Build history of the part. All positions in model axes, mm. A direction names the side the tool comes from. Give positions to 0.01 mm unless a question says otherwise; leave off trailing zeros. Loops run counter-clockwise (first coordinate to the right, second up) from the corner with the lowest first, then second, coordinate; pieces in that order, holes last. Notation, with made-up numbers: (45, 20) - (92, 20) arc R21 ccw to (92, 49) - close; hole circle Ø8 at (-4, -36.5). An arc over 180 degrees is marked (long way). Return JSON: item names as keys, results as strings. Group by question number.
1) Slice it at D-D (x = 4.5). List the corners of the cut face in (y, z), and give its area (3 significant figures).
2) 3-axis set-ups, long thin cutter, end or side, ignore diameter. For faces 1 (the face through (-3.86, 1.22, 0.33)), 2 (the face through (0, 0.25, -5)), 3 (the face through (0, -0.25, -5)), 4 (the face through (0, -0.25, 5)), 5 (the face through (-0.14, 1.55, 0.03)): which of +Z, -Z, +X, -X, +Y, -Y reach the whole face in a straight line?
3) Slice it at B-B (z = 0). List the corners of the cut face in (x, y).
4) Slice it at C-C (y = -0.65). List the corners of the cut face in (x, z).
5) Drop flat-ended pins along their axis: pin 1 (6.5 mm diameter, centred on x = 2.5, z = -5, fed in from +Y); pin 2 (9.5 mm diameter, centred on x = 2, z = 8, fed in from -Y); pin 3 (1 mm diameter, centred on x = -3, y = 0, fed in from +Z). Give the stop position or say it passes through.
6) Drill centre lines: probe 1 along X at (y, z) = (1.3, 0); probe 2 along Z at (x, y) = (1.5, 0.05); probe 3 along Y at (x, z) = (3.5, 0). Where is each one in solid material? Low to high. Write a range as from..to.
7) Slice it at A-A (x = 0). List the corners of the cut face in (y, z).
8) Mould opens along X. For faces 6 (the face through (0, 0.25, 5)), 7 (the face through (-9.865, -0.108, -1.3)), 8 (the face through (4.74, 1.22, 0.33)) say: released by +X, released by -X, zero draft, split by the parting line, or undercut.
Autodesk Inventor part; units mm, degrees
ref_plane "YZ Plane" through (0, 0, 0) normal (1, 0, 0) x (0, 1, 0)
ref_plane "XZ Plane" through (0, 0, 0) normal (0, 1, 0) x (-1, 0, 0)
ref_plane "XY Plane" through (0, 0, 0) normal (0, 0, 1) x (1, 0, 0)
sketch "Sketch1" plane through (0, 0, 0) normal (1, 0, 0) x (0, 1, 0)
  line L0 (-0.25, 9.95) -> (0.25, 9.95)
  line L1 (0.25, -9.95) -> (-0.25, -9.95)
  line L2 (-0.25, 9.95) -> (0.25, -9.95) construction
  line L3 (0.25, 9.95) -> (-0.25, -9.95) construction
  circle A0 centre (0, 0) radius 1.05
  line L4 (0.25, 9.95) -> (0.25, 1.5297)
  line L5 (0.25, -1.5297) -> (0.25, -9.95)
  line L6 (-0.25, -9.95) -> (-0.25, -1.5297)
  line L7 (-0.25, 1.5297) -> (-0.25, 9.95)
  arc A1 (0.25, -1.5297) -> (0.25, 1.5297) centre (0, 0) ccw
  arc A2 (-0.25, 1.5297) -> (-0.25, -1.5297) centre (0, 0) ccw
  dimension "d0" = 0.5
  dimension "d1" = 19.9
  dimension "d3" = 2.1
  dimension "d4" = 0.5
extrude "Extrusion1" add sketch "Sketch1" along normal mid plane 19.9
sketch "Sketch2" plane through (0, 0, 0) normal (0, 1, 0) x (-1, 0, 0)
  circle A0 centre (0, 0) radius 9.95
  circle A1 centre (-4.3, 0) radius 0.55
  line L0 (9.95, 1.5297) -> (-9.95, 1.5297)
  line L1 (0, 1.5297) -> (0, -1.5297)
  line L2 (-9.95, -1.5297) -> (9.95, -1.5297)
  circle A2 centre (4.3, 0) radius 0.55
  dimension "d7" = 19.9
  dimension "d10" = 1.1
  dimension "d11" = 7.5
extrude "Extrusion2" cut sketch "Sketch2" along normal mid plane 10 keep common part
properties part number "flap"
Results:
{
 "1": {"outline": "(-1.46, -0.51) arc R1.55 ccw to (-0.25, -1.53) - (-0.25, -8.87) - (0.25, -8.87) - (0.25, -1.53) arc R1.55 ccw to (1.46, -0.51) - (0.92, -0.51) arc R1.05 cw to (-0.92, -0.51) - close; (-1.46, 0.51) - (-0.92, 0.51) arc R1.05 cw to (0.92, 0.51) - (1.46, 0.51) arc R1.55 ccw to (0.25, 1.53) - (0.25, 8.87) - (-0.25, 8.87) - (-0.25, 1.53) arc R1.55 ccw to start", "area": "10.4 mm2"},
 "2": {"face 1": "+Y, -Y", "face 2": "-Z, +X, -X, +Y", "face 3": "-Z, +X, -X, -Y", "face 4": "+Z, +X, -X, -Y", "face 5": "+X, -X, +Y"},
 "3": {"outline": "(-9.95, -1.55) - (-4.85, -1.55) - (-4.85, -1.05) - (-9.95, -1.05) - close; (-9.95, 1.05) - (-4.85, 1.05) - (-4.85, 1.55) - (-9.95, 1.55) - close; (-3.75, -1.55) - (3.75, -1.55) - (3.75, -1.05) - (-3.75, -1.05) - close; (-3.75, 1.05) - (3.75, 1.05) - (3.75, 1.55) - (-3.75, 1.55) - close; (4.85, -1.55) - (9.95, -1.55) - (9.95, -1.05) - (4.85, -1.05) - close; (4.85, 1.05) - (9.95, 1.05) - (9.95, 1.55) - (4.85, 1.55) - close"},
 "4": {"outline": "(-9.92, -0.82) arc R9.95 ccw to (-9.85, -1.41) - (9.85, -1.41) arc R9.95 ccw to (9.92, -0.82) - close; (-9.92, 0.82) - (9.92, 0.82) arc R9.95 ccw to (9.85, 1.41) - (-9.85, 1.41) arc R9.95 ccw to start"},
 "5": {"pin 1": "y = 0.25", "pin 2": "y = -0.25", "pin 3": "z = 9.63"},
 "6": {"probe 1": "-9.95..-4.85, -3.75..3.75, 4.85..9.95", "probe 2": "-9.84..-1.05, 1.05..9.84", "probe 3": "-1.55..-1.05, 1.05..1.55"},
 "7": {"outline": "(-0.25, -9.95) - (0.25, -9.95) - (0.25, -1.53) arc R1.55 ccw to (0.25, 1.53) - (0.25, 9.95) - (-0.25, 9.95) - (-0.25, 1.53) arc R1.55 ccw to (-0.25, -1.53) - close; hole circle Ø2.1 at (0, 0)"},
 "8": {"face 6": "zero draft", "face 7": "split by the parting line", "face 8": "undercut"}
}
